from build123d import *

# Parameters (mm, degrees)
EXTRUDE1_START   = -15.478468141
EXTRUDE1_DEPTH   = 2.38125
EXTRUDE1_START_2 = 9.127781859
EXTRUDE1_2_DEPTH = 2.38125
EXTRUDE1_START_3 = -13.097218141
EXTRUDE1_3_DEPTH = 22.225
EXTRUDE2_DEPTH   = 2.38125


# Read off the part's stored shape, not the designer's step: Extrude1
with BuildPart() as part:
    # Extrude1 outline → Extrude1 (new body)
    with BuildSketch(Plane.YZ.offset(EXTRUDE1_START)):
        Polygon((863.6, 0), (863.6, -40.573158736), (920.75, -40.682134014), (920.75, 0), align=None)
    extrude(amount=EXTRUDE1_DEPTH)



with BuildPart() as body_2:
    # Extrude1 2 outline → Extrude1 2 (new body)
    with BuildSketch(Plane.YZ.offset(EXTRUDE1_START_2)):
        Polygon((863.6, 0), (863.6, -40.573158736), (920.75, -40.682134014), (920.75, 0), align=None)
    extrude(amount=EXTRUDE1_2_DEPTH)


with BuildPart() as part_1:
    add(part.part)

    add(body_2.part)  # Extrude1 3 merges body 2
    # Extrude1 3 outline → Extrude1 3 (add)
    with BuildSketch(Plane.YZ.offset(EXTRUDE1_START_3)):
        Polygon((865.98125, 0), (863.6, 0), (863.6, -40.573158736), (865.98125, -40.577699373), align=None)
    extrude(amount=EXTRUDE1_3_DEPTH)

    # Sketch2 → Extrude2 (add)
    with BuildSketch(Plane.XY):
        Polygon((18.652781859, 920.75), (9.127781859, 920.75), (9.127781859, 865.98125), (-13.097218141, 865.98125), (-13.097218141, 920.75), (-22.622218141, 920.75), (-22.622218141, 856.45625), (18.652781859, 856.45625), align=None)
    extrude(amount=EXTRUDE2_DEPTH)


solid = part_1.part
Build history of the part. All positions in model axes, mm. A direction names the side the tool comes from. Give positions to 0.01 mm unless a question says otherwise; leave off trailing zeros. Order: outer loops, then holes, each group sorted by start corner. A loop starts at its lowest first (then second) coordinate and runs counter-clockwise, first axis right, second up. Notation, with made-up numbers: M 14,35 L 18,35 A15 cw 18,48 Z; hole C 83.25,61.25 d1. An arc over 180 degrees is marked long. Put each result on its own line as item: value.
Item 1: Cut at D-D on y = 875. Write the cut outline in (x, z), then the cut area to 3 significant figures.
Results are:
outline: M -22.62,0 L -15.48,0 L -15.48,-40.59 L -13.1,-40.59 L -13.1,2.38 L -22.62,2.38 Z; M 9.13,-40.59 L 11.51,-40.59 L 11.51,0 L 18.65,0 L 18.65,2.38 L 9.13,2.38 Z
area: 239 mm2
Item 2: Drop flat-ended pins along their axis: pin 1 Ø5 at (x, z) = (10, -28) entering from -Y; pin 2 Ø12 at (y, z) = (885.5, -18) entering from -X; pin 3 Ø11 at (x, z) = (-2.5, -12) entering from +Y. Give the stop position or say it passes through.
Results are:
pin 1: y = 863.6
pin 2: x = -15.48
pin 3: y = 865.98
Item 3: Pull direction X, two halves, no side cores. Call faces 4 (the face through (9.128, 894, -19)), 5 (the face through (-2, 865.981, -19)), 6 (the face through (-15.478, 892, -20)), 7 (the face through (18.653, 888, 1)): +X half, -X half, draft (parallel to the pull), parting line (faces both ways), or undercut.
Results are:
face 4: undercut
face 5: undercut
face 6: -X half
face 7: +X half
Item 4: Cut at B-B on y = 901. Write the cut outline in (x, z), then the cut area to 3 significant figures.
Results are:
outline: M -22.62,0 L -15.48,0 L -15.48,-40.64 L -13.1,-40.64 L -13.1,2.38 L -22.62,2.38 Z; M 9.13,-40.64 L 11.51,-40.64 L 11.51,0 L 18.65,0 L 18.65,2.38 L 9.13,2.38 Z
area: 239 mm2
Item 5: Which spindle directions (+Z, -Z, +X, -X, +Y, -Y) get a long thin tool onto all of the face, cutting with end or side? Do faces 1 (the face through (11.509, 892, -20)), 2 (the face through (-13.097, 893, -19)), 3 (the face through (-2, 863.6, -20)). Say none if no direction does.
Results are:
face 1: -Z, +X, +Y, -Y
face 2: +Z, -Z, +Y
face 3: -Z, +X, -X, -Y
Item 6: Cut at A-A on z = -10. Write the cut outline in (x, y), then the cut area to 3 significant figures.
Results are:
outline: M -15.48,863.6 L 11.51,863.6 L 11.51,920.75 L 9.13,920.75 L 9.13,865.98 L -13.1,865.98 L -13.1,920.75 L -15.48,920.75 Z
area: 325 mm2
Item 7: Wall check: probe 1 along X at (y, z) = (886, -23); probe 2 along Y at (x, z) = (-13.5, -20); probe 3 along Z at (x, y) = (-20, 875.5). Give the ranges that are in metal, low to high.
Results are:
probe 1: -15.48 to -13.1, 9.13 to 11.51
probe 2: 863.6 to 920.75
probe 3: 0 to 2.38
Item 8: Cut at C-C on x = 8. Write the cut outline in (y, z), then the cut area to 3 significant figures.
Results are:
outline: M 856.46,0 L 863.6,0 L 863.6,-40.57 L 865.98,-40.58 L 865.98,2.38 L 856.46,2.38 Z
area: 119 mm2
